Work out the finished part from the listing and answer in its coordinate system (mm). A direction names the side the tool comes from. Give positions to 0.01 mm unless a question says otherwise; leave off trailing zeros. Order: outer loops, then holes, each group sorted by start corner. A loop starts at its lowest first (then second) coordinate and runs counter-clockwise, first axis right, second up.
```python
from build123d import *

# Parameters (mm, degrees)
F1_DEPTH = 1.524
F3_DEPTH = 40.132
F5_DEPTH = 2.794
F8_R     = 1.5875
F9_R     = 1.5875
F10_R    = 1.5875
F11_R    = 1.5875


with BuildPart() as f1:
    # F0 (on Right) → F1 (new body)
    with BuildSketch(Plane.YZ):
        with BuildLine():
            ThreePointArc((26.67, 36.195), (25.7400640303, 38.4400640303), (23.495, 39.37))
            Line((23.495, 39.37), (-23.495, 39.37))
            ThreePointArc((-23.495, 39.37), (-25.7400640303, 38.4400640303), (-26.67, 36.195))
            Line((-26.67, 36.195), (-26.67, -36.195))
            ThreePointArc((-26.67, -36.195), (-25.7400640303, -38.4400640303), (-23.495, -39.37))
            Line((-23.495, -39.37), (23.495, -39.37))
            ThreePointArc((23.495, -39.37), (25.7400640303, -38.4400640303), (26.67, -36.195))
            Line((26.67, -36.195), (26.67, 36.195))
        make_face()
    extrude(amount=F1_DEPTH)

    # F2 (on face) → F3 (join)
    with BuildSketch(Plane(origin=(0, 0, 0), x_dir=(0, -1, 0), z_dir=(-1, 0, 0))):
        with BuildLine():
            Line((23.495, 39.37), (-23.495, 39.37))
            ThreePointArc((-23.495, 39.37), (-25.7400640303, 38.4400640303), (-26.67, 36.195))
            Line((-26.67, 36.195), (-26.67, -36.195))
            ThreePointArc((-26.67, -36.195), (-25.7400640303, -38.4400640303), (-23.495, -39.37))
            Line((-23.495, -39.37), (23.495, -39.37))
            ThreePointArc((23.495, -39.37), (25.7400640303, -38.4400640303), (26.67, -36.195))
            Line((26.67, -36.195), (26.67, 36.195))
            ThreePointArc((26.67, 36.195), (25.7400640303, 38.4400640303), (23.495, 39.37))
        make_face()
        with BuildLine():
            ThreePointArc((25.146, -36.2585), (24.6810320151, -37.3810320151), (23.5585, -37.846))
            Line((23.5585, -37.846), (-23.5585, -37.846))
            ThreePointArc((-23.5585, -37.846), (-24.6810320151, -37.3810320151), (-25.146, -36.2585))
            Line((-25.146, -36.2585), (-25.146, 36.2585))
            ThreePointArc((-25.146, 36.2585), (-24.6810320151, 37.3810320151), (-23.5585, 37.846))
            Line((-23.5585, 37.846), (23.5585, 37.846))
            ThreePointArc((23.5585, 37.846), (24.6810320151, 37.3810320151), (25.146, 36.2585))
            Line((25.146, 36.2585), (25.146, -36.2585))
        make_face(mode=Mode.SUBTRACT)
    extrude(amount=F3_DEPTH)

    # F4 (on face) → F5 (join)
    with BuildSketch(Plane.YZ.offset(1.524)):
        with BuildLine():
            ThreePointArc((-26.67, 33.02), (-22.1798719395, 34.8798719395), (-20.32, 39.37))
            Line((-20.32, 39.37), (-23.495, 39.37))
            ThreePointArc((-23.495, 39.37), (-25.7400640303, 38.4400640303), (-26.67, 36.195))
            Line((-26.67, 36.195), (-26.67, 33.02))
        make_face()
    extrude(amount=F5_DEPTH)


with BuildPart() as f6_1:
    # F6: instance of F1
    add(f1.part.mirror(Plane.XY))


with BuildPart() as f1_1:
    add(f1.part)

    add(f6_1.part)  # F7 merges F6_1
    # F7: F6_1, F1 across plane
    add(f6_1.part.mirror(Plane.XZ))
    add(f1.part.mirror(Plane.XZ))

    # F8
    f8_edges = [f1_1.edges().sort_by_distance(p)[0] for p in [
        (1.524, -26.67, 0),
    ]]
    fillet(f8_edges, radius=F8_R)

    # F9
    f9_edges = [f1_1.edges().sort_by_distance(p)[0] for p in [
        (1.524, 0, -39.37),
    ]]
    fillet(f9_edges, radius=F9_R)

    # F10
    f10_edges = [f1_1.edges().sort_by_distance(p)[0] for p in [
        (1.524, 26.67, 0),
    ]]
    fillet(f10_edges, radius=F10_R)

    # F11
    f11_edges = [f1_1.edges().sort_by_distance(p)[0] for p in [
        (1.524, 0, 39.37),
    ]]
    fillet(f11_edges, radius=F11_R)


solid = f1_1.part
```
1. Which of the six approach directions +Z, -Z, +X, -X, +Y, -Y give full straight-line access (tool end or side, diameter ignored) to faces 1 (the face through (-20, 0, -37.846)), 2 (the face through (2.58, -22.23, -34.83)), 3 (the face through (4.318, 24, -36))?
Findings below:
face 1: -X
face 2: +X
face 3: +Z, -Z, +X, +Y, -Y
2. Straight lines are drawn through the part: probe 1 along Y at (x, z) = (-21.5, -6.5); probe 2 along Z at (x, y) = (-38, -9.5); probe 3 along X at (y, z) = (18, 8). For each, find the intervals that lie inside material, in ascending order.
Findings below:
probe 1: y = -26.67 to -25.15, 25.15 to 26.67
probe 2: z = -39.37 to -37.85, 37.85 to 39.37
probe 3: x = 0 to 1.52
3. Given P1, Ø4, axis at y = 11.5, z = -23.5, coming from the -X side; P2, Ø12, axis at y = 2, z = 16, coming from the +X side, each flat-ended and moving along its own axis, determine where each tip first touches the part or whether it passes through.
Findings below:
P1: stops at x = 0
P2: stops at x = 1.52
4. The part is cut by section C-C (z = -1). Write down the section's boundary in (x, y) (1 decimal), then the cut area to 3 significant figures.
Findings below:
outline: (-40.1, -26.7) - (-0.1, -26.7) arc R1.6 ccw to (1.5, -25.1) - (1.5, 25.1) arc R1.6 ccw to (-0.1, 26.7) - (-40.1, 26.7) - (-40.1, 25.1) - (0, 25.1) - (0, -25.1) - (-40.1, -25.1) - close
area: 203 mm2
5. The part is cut by section B-B (y = 6). Write down the section's boundary in (x, z) (1 decimal).
Findings below:
outline: (-40.1, -39.4) - (-0.1, -39.4) arc R1.6 ccw to (1.5, -37.8) - (1.5, 37.8) arc R1.6 ccw to (-0.1, 39.4) - (-40.1, 39.4) - (-40.1, 37.8) - (0, 37.8) - (0, -37.8) - (-40.1, -37.8) - close
